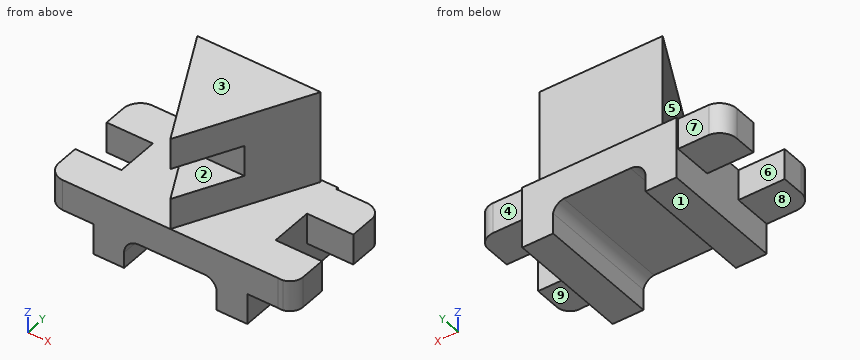
```python
from build123d import *

# Parameters (mm, degrees)
F1_DEPTH  = 25.4
F3_DEPTH  = 25.4
F5_DEPTH  = 25.4
F6_DEPTH  = 25.4
F8_DEPTH  = 25.4
F9_DEPTH  = 25.4
F11_DEPTH = 101.6


with BuildPart() as f1:
    # F0 (on Top) → F1 (new body)
    with BuildSketch(Plane.XY):
        Polygon((50.8, 50.5276115144), (-50.8, 50.5276115144), (0, -49.1656845147), align=None)
    extrude(amount=F1_DEPTH)

    # F2 (on face) → F3 (join)
    with BuildSketch(Plane(origin=(0, 0, 0), x_dir=(1, 0, 0), z_dir=(0, 0, -1))):
        Polygon((0, 0), (-25.0530062986, 0), (-50.8, -50.5276115144), (50.8, -50.5276115144), (25.0530062986, 0), align=None)
    extrude(amount=F3_DEPTH)

    # F4 (on face) → F5 (join)
    with BuildSketch(Plane(origin=(0, 0, -25.4), x_dir=(1, 0, 0), z_dir=(0, 0, -1))):
        Polygon((25.0530062986, 0), (-25.0530062986, 0), (-50.8, -50.5276115144), (50.8, -50.5276115144), align=None)
    extrude(amount=F5_DEPTH)

    # F4 (on face) → F6 (join)
    with BuildSketch(Plane(origin=(0, 0, -25.4), x_dir=(1, 0, 0), z_dir=(0, 0, -1))):
        Polygon((0, 49.1656845147), (-25.0530062986, 0), (25.0530062986, 0), align=None)
    extrude(amount=F6_DEPTH)

    # F7 (on face) → F8 (join)
    with BuildSketch(Plane(origin=(0, 0, -50.8), x_dir=(1, 0, 0), z_dir=(0, 0, -1))):
        with BuildLine():
            ThreePointArc((92.8366021578, 49.1656845147), (90.8683010789, 49.3477316598), (88.9, 49.1656845147))
            Line((88.9, 49.1656845147), (92.8366021578, 49.1656845147))
        make_face()
        Polygon((-50.8, -50.5276115144), (0, -50.5276115144), (50.8, -50.5276115144), (0, 49.1656845147), align=None)
        with BuildLine():
            Line((0, 49.1656845147), (50.8, -50.5276115144))
            Line((50.8, -50.5276115144), (88.9, -50.5276115144))
            ThreePointArc((88.9, -50.5276115144), (96.9463521433, -47.7655661288), (101.6, -40.6440326455))
            Line((101.6, -40.6440326455), (101.6, -17.8896365181))
            Line((101.6, -17.8896365181), (63.5, -17.8896365181))
            Line((63.5, -17.8896365181), (63.5, 17.4156845147))
            Line((63.5, 17.4156845147), (101.6, 17.4156845147))
            Line((101.6, 17.4156845147), (101.6, 38.6160327387))
            ThreePointArc((101.6, 38.6160327387), (99.1233775867, 45.4733699467), (92.8366021578, 49.1656845147))
            Line((92.8366021578, 49.1656845147), (88.9, 49.1656845147))
            Line((88.9, 49.1656845147), (0, 49.1656845147))
        make_face()
    extrude(amount=F8_DEPTH)

    # F7 (on face) → F9 (join)
    with BuildSketch(Plane(origin=(0, 0, -50.8), x_dir=(1, 0, 0), z_dir=(0, 0, -1))):
        with BuildLine():
            Line((-88.9, -50.5276115144), (-50.8, -50.5276115144))
            Line((-50.8, -50.5276115144), (0, 49.1656845147))
            Line((0, 49.1656845147), (-88.9, 49.1656845147))
            ThreePointArc((-88.9, 49.1656845147), (-97.9199978671, 45.0034008683), (-101.6, 35.7761287374))
            Line((-101.6, 35.7761287374), (-101.6, 17.4156845147))
            Line((-101.6, 17.4156845147), (-63.5, 17.4156845147))
            Line((-63.5, 17.4156845147), (-63.5, -17.8896365181))
            Line((-63.5, -17.8896365181), (-101.6, -17.8896365181))
            Line((-101.6, -17.8896365181), (-101.6, -36.3230473445))
            ThreePointArc((-101.6, -36.3230473445), (-97.9620426965, -45.8501093688), (-88.9, -50.5276115144))
        make_face()
    extrude(amount=F9_DEPTH)

    # F10 (on face) → F11 (join)
    with BuildSketch(Plane.XZ.offset(49.1656845147)):
        with BuildLine():
            Line((-63.5, -50.8), (-63.5, -76.2))
            Line((-63.5, -76.2), (-63.5, -101.6))
            Line((-63.5, -101.6), (-38.1, -101.6))
            Line((-38.1, -101.6), (-38.1, -88.9))
            ThreePointArc((-38.1, -88.9), (-38.1009544934, -88.7452450805), (-38.1, -88.5904901609))
            ThreePointArc((-38.1, -88.5904901609), (-34.4176212284, -79.86523026), (-25.6851438653, -76.2))
            ThreePointArc((-25.6851438653, -76.2), (-25.5550347378, -76.1993253249), (-25.4249256104, -76.2))
            Line((-25.4249256104, -76.2), (26.2085422873, -76.2))
            ThreePointArc((26.2085422873, -76.2), (27.7959470911, -76.0795943408), (29.3833518949, -76.2))
            ThreePointArc((29.3833518949, -76.2), (35.0360054884, -78.9657015641), (38.1, -84.4623856029))
            ThreePointArc((38.1, -84.4623856029), (38.320168092, -86.6038153417), (38.1, -88.7452450805))
            Line((38.1, -88.7452450805), (38.1, -101.6))
            Line((38.1, -101.6), (63.5, -101.6))
            Line((63.5, -101.6), (63.5, -76.2))
            Line((63.5, -76.2), (63.5, -50.8))
            Line((63.5, -50.8), (-63.5, -50.8))
        make_face()
        with BuildLine():
            ThreePointArc((-38.1, -88.5904901609), (-38.1009544934, -88.7452450805), (-38.1, -88.9))
            Line((-38.1, -88.9), (-38.1, -88.5904901609))
        make_face()
        with BuildLine():
            ThreePointArc((-25.4249256104, -76.2), (-25.5550347378, -76.1993253249), (-25.6851438653, -76.2))
            Line((-25.6851438653, -76.2), (-25.4249256104, -76.2))
        make_face()
        with BuildLine():
            Line((38.1, -84.4623856029), (38.1, -88.7452450805))
            ThreePointArc((38.1, -88.7452450805), (38.320168092, -86.6038153417), (38.1, -84.4623856029))
        make_face()
        with BuildLine():
            ThreePointArc((29.3833518949, -76.2), (27.7959470911, -76.0795943408), (26.2085422873, -76.2))
            Line((26.2085422873, -76.2), (29.3833518949, -76.2))
        make_face()
    extrude(amount=-F11_DEPTH)


solid = f1.part
```
Design review of the part built by this model. Coordinates are the model's own, in mm. Face numbers are marked on the shaded views. A direction names the side the tool comes from. Give positions to 0.01 mm unless a question says otherwise; leave off trailing zeros. Order: outer loops, then holes, each group sorted by start corner. A loop starts at its lowest first (then second) coordinate and runs counter-clockwise, first axis right, second up. Notation, with made-up numbers: M 20.5,-27.75 L 37.5,-27.75 A32 ccw 37.5,9.25 Z; hole C 36.5,58.5 d9. An arc over 180 degrees is marked long. One line per question, with ' | ' between items. Start each with the question number.
Q1. For L1, parallel to X at y = -40, z = -90; L2, parallel to Z at x = -5, y = -35.5; L3, parallel to Y at x = 2.5, z = -72.5, list the stretches that pass through material, from the lowest coordinate up. Write a range as [from, to].
Q2. The part is to be moulded in two halves that separate along Z. For the marked faces 1, 2, 3 and 4, say which applies: +Z half, -Z half, draft (parallel to the pull), parting line (faces both ways), or undercut.
Q3. We need section B-B (y = -29). Write out the cut boundary in (x, z), plus the area to 3 significant figures.
Q4. We need section D-D (x = 48). Write out the cut boundary in (y, z), plus the area to 3 significant figures.
Q5. We need section C-C (z = -62.5). Write out the cut boundary in (x, y), plus the area to 3 significant figures.
Q6. Machinability: for the marked faces 5, 6, 7, 8 and 9, which of the approach directions +Z, -Z, +X, -X, +Y, -Y give a long, thin tool a straight path to every point of the face, cutting with its end or side? Answer none if there is none.
Q7. We need section A-A (x = -73.5). Write out the cut boundary in (y, z), plus the area to 3 significant figures.
Q8. For pin 1 Ø5 at (x, y) = (58.5, -9) entering from +Z; pin 2 Ø5 at (y, z) = (25.5, -91) entering from -X; pin 3 Ø23 at (x, z) = (0.5, 2) entering from +Y; pin 4 Ø10 at (x, z) = (-16.5, -50.5) entering from +Y, all flat-tipped, find the tip position at first contact; note any pin that passes through.
Returned:
1) L1: [-63.5, -38.1], [38.1, 63.5] | L2: [-76.2, -25.4], [0, 25.4] | L3: [-49.17, 52.43]
2) face 1: -Z half | face 2: undercut | face 3: +Z half | face 4: draft
3) outline: M -101.6,-76.2 L -63.5,-76.2 L -63.5,-101.6 L -38.1,-101.6 L -38.1,-88.59 A12.55 cw -25.69,-76.2 L 29.38,-76.2 A10.52 cw 38.1,-84.46 L 38.1,-101.6 L 63.5,-101.6 L 63.5,-76.2 L 101.6,-76.2 L 101.6,-50.8 L 10.28,-50.8 L 10.28,-25.4 L -10.28,-25.4 L -10.28,-50.8 L -101.6,-50.8 Z; M -10.28,0 L 10.28,0 L 10.28,25.4 L -10.28,25.4 Z | area: 7,550 mm2
4) outline: M -49.17,-101.6 L 52.43,-101.6 L 52.43,-50.8 L 50.53,-50.8 L 50.53,25.4 L 45.03,25.4 L 45.03,-50.8 L -49.17,-50.8 Z | area: 5,580 mm2
5) outline: M -101.6,-35.78 A13.41 ccw -88.9,-49.17 L 88.9,-49.17 A10.73 ccw 101.6,-38.62 L 101.6,-17.42 L 63.5,-17.42 L 63.5,17.89 L 101.6,17.89 L 101.6,40.64 A13.1 ccw 88.9,50.53 L 63.5,50.53 L 63.5,52.43 L -63.5,52.43 L -63.5,50.53 L -88.9,50.53 A14.29 ccw -101.6,36.32 L -101.6,17.89 L -63.5,17.89 L -63.5,-17.42 L -101.6,-17.42 Z | area: 17,700 mm2
6) face 5: +Z, -X, -Y | face 6: +Z, -Z, -X | face 7: +Z, -Z, -X, +Y | face 8: -Z, -X, +Y, -Y | face 9: -Z, +X, +Y, -Y
7) outline: M -49.17,-76.2 L -17.42,-76.2 L -17.42,-50.8 L -49.17,-50.8 Z; M 17.89,-76.2 L 50.53,-76.2 L 50.53,-50.8 L 17.89,-50.8 Z | area: 1,640 mm2
8) pin 1: z = -50.8 | pin 2: x = -63.5 | pin 3: y = 50.53 | pin 4: y = 52.43
